Can you work these out from the drawing? Everything is in mm from the part's minimum corner. A direction names the side the tool comes from. Coordinates: 2 decimals unless noted, no trailing zeros. Order: outer loops, then holes, each group sorted by start corner. A loop starts at its lowest first (then second) coordinate and runs counter-clockwise, first axis right, second up. Notation, with made-up numbers: (59, 43.5) - (77, 43.5) arc R26 cw to (77, 60.5) - close; hole circle Ø4 at (75, 65.25). An arc over 180 degrees is marked (long way). Use a Markdown table: item, result. Add a question column.
(1) I want a section at D-D (x = 30). List the corners of the cut face in (y, z) for me, and give its area (3 significant figures).
(2) If I drill on L1, parallel to X at y = 1.25, z = 22.75; L2, parallel to X at y = 5.25, z = 9.75; L3, parallel to Y at x = 46.5, z = 18.5, over which ranges is the centre line in solid material (lowest first)? Write a range as [from, to].
(3) I want a section at A-A (x = 47.25). List the corners of the cut face in (y, z) for me.
(4) I want a section at B-B (y = 6.25). List the corners of the cut face in (x, z) for me, and give its area (3 significant figures).
(5) On a 3-axis mill with a long thin cutter (end or side, diameter ignored), from which of +Z, -Z, +X, -X, +Y, -Y can I reach the whole of each face in a straight line? I mean the marked faces 1, 2 and 3. Say none if no direction works.
(6) For pin 1 Ø1 at (x, y) = (23, 5.5) entering from +Z; pin 2 Ø3.5 at (x, y) = (3, 4) entering from -Z; pin 3 Ø7.5 at (y, z) = (10, 12.5) entering from +X; pin 4 Ø2.5 at (x, y) = (47, 7) entering from +Z, each with a flat end and sliding along its axis, tell me the tip position at first contact or that it passes through.
(7) I want a section at C-C (z = 14.5). List the corners of the cut face in (x, y) for me, and give its area (3 significant figures).
(8) We'd pull the mould along X, two halves only. Please class the marked faces 4, 5 and 6: pulls with the +X half, pulls with the -X half, needs draft (parallel to the pull), parting line crosses it, or undercut.
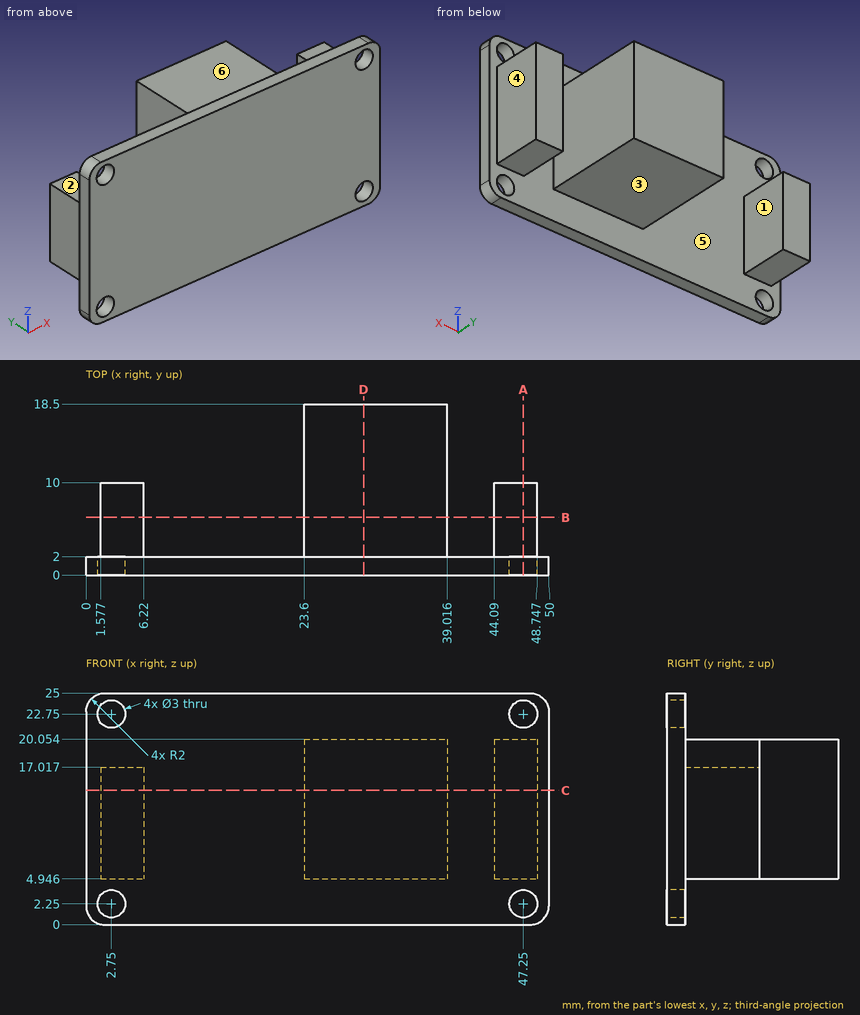
Answers follow:
| question | item | result |
|---|---|---|
| 1 | outline | (0, 0) - (2, 0) - (2, 4.95) - (18.5, 4.95) - (18.5, 20.05) - (2, 20.05) - (2, 25) - (0, 25) - close |
| 1 | area | 299 mm² |
| 2 | L1 | x = [0, 1.25], [4.25, 45.75], [48.75, 50] |
| 2 | L2 | x = [1.58, 6.22], [23.6, 39.02], [44.09, 48.75] |
| 2 | L3 | y = [0, 10] |
| 3 | outline | (0, 0) - (2, 0) - (2, 0.75) - (0, 0.75) - close; (0, 3.75) - (2, 3.75) - (2, 4.95) - (10, 4.95) - (10, 20.05) - (2, 20.05) - (2, 21.25) - (0, 21.25) - close; (0, 24.25) - (2, 24.25) - (2, 25) - (0, 25) - close |
| 4 | outline | (1.58, 4.95) - (6.22, 4.95) - (6.22, 17.02) - (1.58, 17.02) - close; (23.6, 4.95) - (39.02, 4.95) - (39.02, 20.05) - (23.6, 20.05) - close; (44.09, 4.95) - (48.75, 4.95) - (48.75, 20.05) - (44.09, 20.05) - close |
| 4 | area | 359 mm² |
| 5 | face 1 | +Z, -Z, +Y |
| 5 | face 2 | +Z, -X, +Y |
| 5 | face 3 | -Z, +X, -X, +Y |
| 6 | pin 1 | passes through |
| 6 | pin 2 | stops at z = 4.95 |
| 6 | pin 3 | stops at x = 48.75 |
| 6 | pin 4 | stops at z = 20.05 |
| 7 | outline | (0, 0) - (50, 0) - (50, 2) - (48.75, 2) - (48.75, 10) - (44.09, 10) - (44.09, 2) - (39.02, 2) - (39.02, 18.5) - (23.6, 18.5) - (23.6, 2) - (6.22, 2) - (6.22, 10) - (1.58, 10) - (1.58, 2) - (0, 2) - close |
| 7 | area | 429 mm² |
| 8 | face 4 | pulls with the +X half |
| 8 | face 5 | undercut |
| 8 | face 6 | needs draft |
